Design review of the part built by this model. Coordinates are the model's own, in mm. A direction names the side the tool comes from. Coordinates: 2 decimals unless noted, no trailing zeros. Write each loop counter-clockwise with the first axis right and the second up, starting at its lowest first coordinate (ties: lowest second). Pieces come first, ordered by that corner, then holes. Notation, with made-up numbers: M 55.25,6.5 L 83.25,6.5 A16 ccw 83.25,27.5 Z; hole C 6,-6.75 d9. An arc over 180 degrees is marked long. Write item = value, one per line.
```python
from build123d import *

# Parameters (mm, degrees)
SKETCH2_W           = 38.1
SKETCH2_H           = 19.05
SKETCH2_W_2         = 34.798
SKETCH2_H_2         = 15.748
BOSS_EXTRUDE1_DEPTH = 203.2
SKETCH3_R           = 1.016
CUT_EXTRUDE1_DEPTH  = 39.1
CUT_EXTRUDE2_REACH  = 21.05
SKETCH6_R           = 1.016


with BuildPart() as part:
    # Sketch2 → Boss-Extrude1 (new body)
    with BuildSketch(Plane.XY):
        Rectangle(SKETCH2_W, SKETCH2_H)
        Rectangle(SKETCH2_W_2, SKETCH2_H_2, mode=Mode.SUBTRACT)
    extrude(amount=BOSS_EXTRUDE1_DEPTH)

    # Sketch3 → Cut-Extrude1 (cut, through all)
    with BuildSketch(Plane(origin=(19.05, 0, 0), x_dir=(0, 0, -1), z_dir=(1, 0, 0))):
        with Locations((-196.85, 0)):
            Circle(SKETCH3_R)
        with Locations((-156.21, 0)):
            Circle(SKETCH3_R)
    extrude(amount=-CUT_EXTRUDE1_DEPTH, mode=Mode.SUBTRACT)

    # Sketch6 → Cut-Extrude2 (cut, up to next)
    with BuildSketch(Plane(origin=(0, 9.525, 0), x_dir=(1, 0, 0), z_dir=(0, 1, 0)), mode=Mode.PRIVATE) as cut_extrude2_sk1:
        with Locations((0, -12.7)):
            Circle(SKETCH6_R)
    cut_extrude2_tool1 = extrude(cut_extrude2_sk1.sketch, amount=-CUT_EXTRUDE2_REACH, mode=Mode.PRIVATE) & part.part
    add(cut_extrude2_tool1.solids().sort_by_distance((0, 9.525, 12.7))[0], mode=Mode.SUBTRACT)
    # Sketch6 → Cut-Extrude2 (cut, up to next)
    with BuildSketch(Plane(origin=(0, 9.525, 0), x_dir=(1, 0, 0), z_dir=(0, 1, 0)), mode=Mode.PRIVATE) as cut_extrude2_sk2:
        with Locations((0, -44.704)):
            Circle(SKETCH6_R)
    cut_extrude2_tool2 = extrude(cut_extrude2_sk2.sketch, amount=-CUT_EXTRUDE2_REACH, mode=Mode.PRIVATE) & part.part
    add(cut_extrude2_tool2.solids().sort_by_distance((0, 9.525, 44.704))[0], mode=Mode.SUBTRACT)


solid = part.part
```
Q1. Machinability: for faces 1 (the flat face through (-1.5, -8.4, 0)), 2 (the flat face through (0, -7.874, 100)), which of the approach directions +Z, -Z, +X, -X, +Y, -Y give a long, thin tool a straight path to every point of the face, cutting with its end or side? Answer none if there is none.
Check result:
face_1 = -Z, +X, -X, +Y, -Y
face_2 = +Z, -Z
Q2. The part is to be moulded in two halves that separate along X. For faces 3 (the flat face through (19.05, 0, 100)), 4 (the flat face through (17.399, 0, 100)), 5 (the flat face through (0, 9.525, 100)), say which applies: +X half, -X half, draft (parallel to the pull), parting line (faces both ways), or undercut.
Check result:
face_3 = +X half
face_4 = undercut
face_5 = draft
Q3. For P1, Ø6, axis at x = 9.5, y = -6.5, coming from the -Z side; P2, Ø1.8, axis at y = 0, z = 156.21, coming from the +X side, all flat-tipped, find the tip position at first contact; note any pin that passes through.
Check result:
P1 = 0
P2 = through
Q4. Consider section B-B, the plane z = 60.5. State the section outline as (x, y) points (3 decimals), and give its area (3 significant figures).
Check result:
outline = M -19.05,-9.525 L 19.05,-9.525 L 19.05,9.525 L -19.05,9.525 Z; hole M -17.399,-7.874 L 17.399,-7.874 L 17.399,7.874 L -17.399,7.874 Z
area = 178 mm²
Q5. Consider section A-A, the plane x = -9. State the section outline as (y, z) points (3 decimals).
Check result:
outline = M -9.525,0 L -7.874,0 L -7.874,203.2 L -9.525,203.2 Z; M 7.874,0 L 9.525,0 L 9.525,203.2 L 7.874,203.2 Z
Q6. Wall thickness on line 1 (Y direction, x = 18.15, z = 196.85) (3 decimals); line 2 (X direction, y = 3.5, z = 120); line 3 (Y direction, x = 12.5, z = 90) (3 decimals): over which ranges is each line inside the solid? List them lowest first.
Check result:
line_1 = -9.525 to -1.016, 1.016 to 9.525
line_2 = -19.05 to -17.4, 17.4 to 19.05
line_3 = -9.525 to -7.874, 7.874 to 9.525
